from build123d import *

# Parameters (mm, degrees)
F0_W     = 42.3
F0_H     = 42.3
F1_DEPTH = 59
F2_R     = 11
F3_DEPTH = 2
F4_R     = 2.5
F5_DEPTH = 22
F7_DEPTH = 15
F9_DEPTH = 4.5


with BuildPart() as f1:
    # F0 (on Front) → F1 (new body)
    with BuildSketch(Plane.XZ):
        Rectangle(F0_W, F0_H)
    extrude(amount=F1_DEPTH)

    # F2 (on face) → F3 (join)
    with BuildSketch(Plane.XZ.offset(59)):
        Circle(F2_R)
    extrude(amount=F3_DEPTH)

    # F4 (on face) → F5 (join)
    with BuildSketch(Plane.XZ.offset(61)):
        Circle(F4_R)
    extrude(amount=F5_DEPTH)

    # F6 (on face) → F7 (cut)
    with BuildSketch(Plane.XZ.offset(83)):
        with BuildLine():
            ThreePointArc((0, 2.5), (-0.790569, 2.371708), (-1.5, 2))
            Line((-1.5, 2), (0, 2))
            Line((0, 2), (0, 2.5))
        make_face()
        with BuildLine():
            Line((0, 2.5), (0, 2))
            Line((0, 2), (1.5, 2))
            ThreePointArc((1.5, 2), (0.790569, 2.371708), (0, 2.5))
        make_face()
    extrude(amount=-F7_DEPTH, mode=Mode.SUBTRACT)

    # F8 (on face) → F9 (cut)
    with BuildSketch(Plane.XZ.offset(59)):
        with BuildLine():
            ThreePointArc((16.75, 15.5), (15.5, 16.75), (14.25, 15.5))
            Line((14.25, 15.5), (15.5, 15.5))
            Line((15.5, 15.5), (15.5, 14.25))
            ThreePointArc((15.5, 14.25), (16.383883, 14.616117), (16.75, 15.5))
        make_face()
        with BuildLine():
            Line((15.5, 15.5), (14.25, 15.5))
            ThreePointArc((14.25, 15.5), (14.616117, 14.616117), (15.5, 14.25))
            Line((15.5, 14.25), (15.5, 15.5))
        make_face()
        with BuildLine():
            Line((-15.5, 14.25), (-15.5, 15.5))
            Line((-15.5, 15.5), (-14.25, 15.5))
            ThreePointArc((-14.25, 15.5), (-16.383883, 16.383883), (-15.5, 14.25))
        make_face()
        with BuildLine():
            Line((-14.25, 15.5), (-15.5, 15.5))
            Line((-15.5, 15.5), (-15.5, 14.25))
            ThreePointArc((-15.5, 14.25), (-14.616117, 14.616117), (-14.25, 15.5))
        make_face()
        with BuildLine():
            Line((-15.5, -15.5), (-15.5, -14.25))
            ThreePointArc((-15.5, -14.25), (-16.383883, -16.383883), (-14.25, -15.5))
            Line((-14.25, -15.5), (-15.5, -15.5))
        make_face()
        with BuildLine():
            ThreePointArc((-14.25, -15.5), (-14.616117, -14.616117), (-15.5, -14.25))
            Line((-15.5, -14.25), (-15.5, -15.5))
            Line((-15.5, -15.5), (-14.25, -15.5))
        make_face()
        with BuildLine():
            Line((15.5, -15.5), (15.5, -14.25))
            ThreePointArc((15.5, -14.25), (14.616117, -14.616117), (14.25, -15.5))
            Line((14.25, -15.5), (15.5, -15.5))
        make_face()
        with BuildLine():
            ThreePointArc((16.75, -15.5), (16.383883, -14.616117), (15.5, -14.25))
            Line((15.5, -14.25), (15.5, -15.5))
            Line((15.5, -15.5), (14.25, -15.5))
            ThreePointArc((14.25, -15.5), (15.5, -16.75), (16.75, -15.5))
        make_face()
    extrude(amount=-F9_DEPTH, mode=Mode.SUBTRACT)


solid = f1.part
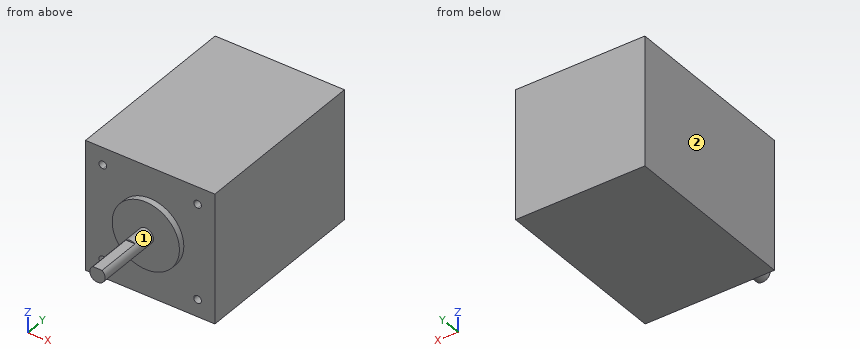
Verification items for the finished model (mm, model axes). Face numbers are marked on the shaded views. A direction names the side the tool comes from. Coordinates: 2 decimals unless noted, no trailing zeros. Loops run counter-clockwise (first coordinate to the right, second up) from the corner with the lowest first, then second, coordinate; pieces in that order, holes last. Notation, with made-up numbers: (54.5, 56) -> (67.5, 56) arc R31 cw to (67.5, 92) -> close; hole circle Ø3 at (-12, 56.25). An arc over 180 degrees is marked (long way). Answer as a JSON object with one key per item and string values. Group by question number.
Item 1: Sectioned sample at C-C on y = -74.5. Record the boundary of the cut face in (x, z).
Item 2: Depth check by flat-ended pin: pin 1 (4 mm diameter, centred on x = -15.5, z = -15.5, fed in from -Y); pin 2 (3 mm diameter, centred on x = 3.5, y = -74, fed in from +Z); pin 3 (2 mm diameter, centred on x = -15.5, z = 15.5, fed in from -Y). Enter the tip coordinate at first touch or a pass-through.
Item 3: Sectioned sample at D-D on z = -9. Record the boundary of the cut face in (x, y).
Item 4: Sectioned sample at A-A on x = 0. Record the boundary of the cut face in (y, z).
Item 5: Sectioned sample at B-B on z = 0. Record the boundary of the cut face in (x, y).
Item 6: Scan lines: probe 1 along Z at (x, y) = (-15.5, -57.95); probe 2 along X at (y, z) = (-55, -15). Record each from-to range of solid material in increasing order.
Item 7: Tool access check on the marked faces 1 and 2. Record the directions out of +Z, -Z, +X, -X, +Y, -Y that give a thin tool (end or side, any length) a straight path to the whole face; none if there is none.
Evaluation:
{
 "1": {"outline": "(-1.5, 2) arc R2.5 ccw (long way) to (1.5, 2) -> close"},
 "2": {"pin 1": "stops at y = -59", "pin 2": "stops at z = 1.5", "pin 3": "stops at y = -54.5"},
 "3": {"outline": "(-21.15, -59) -> (-6.32, -59) -> (-6.32, -61) -> (6.32, -61) -> (6.32, -59) -> (21.15, -59) -> (21.15, 0) -> (-21.15, 0) -> close"},
 "4": {"outline": "(-83, -2.5) -> (-61, -2.5) -> (-61, -11) -> (-59, -11) -> (-59, -21.15) -> (0, -21.15) -> (0, 21.15) -> (-59, 21.15) -> (-59, 11) -> (-61, 11) -> (-61, 2.5) -> (-68, 2.5) -> (-68, 2) -> (-83, 2) -> close"},
 "5": {"outline": "(-21.15, -59) -> (-11, -59) -> (-11, -61) -> (-2.5, -61) -> (-2.5, -83) -> (2.5, -83) -> (2.5, -61) -> (11, -61) -> (11, -59) -> (21.15, -59) -> (21.15, 0) -> (-21.15, 0) -> close"},
 "6": {"probe 1": "z = -21.15 to -16.75, -14.25 to 14.25, 16.75 to 21.15", "probe 2": "x = -21.15 to -16.65, -14.35 to 14.35, 16.65 to 21.15"},
 "7": {"face 1": "-Y", "face 2": "+Z, -Z, -X, +Y, -Y"}
}
